Geometry: see drawing. Coordinates: mm, zero at the bounding-box minimum. Round coordinates to 2 decimals unless told otherwise and drop trailing zeros. Order: outer loops, then holes, each group sorted by start corner. A loop starts at its lowest first (then second) coordinate and runs counter-clockwise, first axis right, second up. Notation, with made-up numbers: (30.25, 73.25) -> (36.25, 73.25) arc R22 ccw to (36.25, 108.25) -> close; hole circle Ø4 at (-13, 87). An arc over 180 degrees is marked (long way). Answer as CSV lines item,"result". Start each with the question number.
(1) Section query A-A (y = 0.9). Output: boundary loops of the cut face in (x, z).
(2) Section query B-B (x = 54). Output: boundary loops of the cut face in (y, z).
(3) Contact query for flat-ended pins moving along their axis: P1, Ø0.9, axis at y = 1, z = 81.5, coming from the +X side; P2, Ø1.5, axis at x = 55, y = 1.5, coming from the -Z side. Output: stop coordinate, or through.
(4) Section query C-C (z = 18.5). Output: boundary loops of the cut face in (x, y), plus the area to 3 significant figures.
(5) Line query: line 1 along Z through (x, y) = (55.5, 1.65); line 2 along X through (y, z) = (2.6, 14); line 3 along X through (y, z) = (0.2, 61.5) (3 decimals). Output: solid intervals per line, ascending. Write a range as from..to.
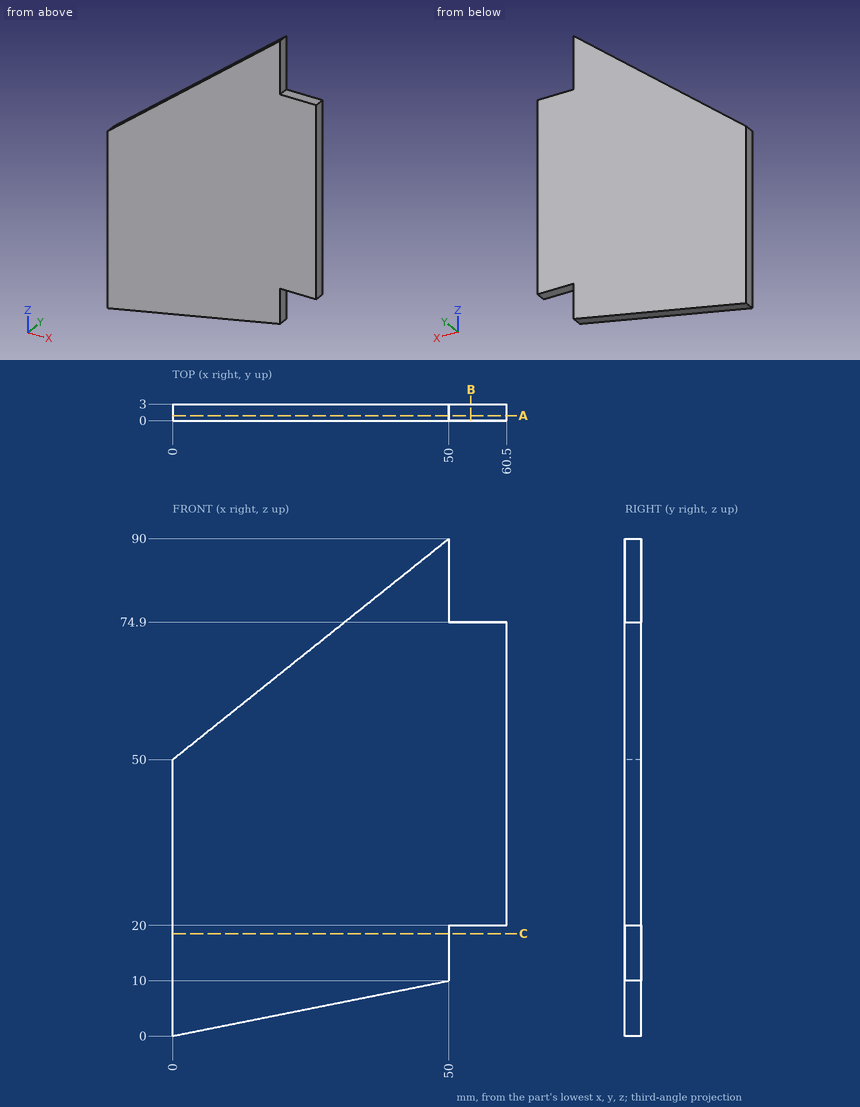
Answer block:
1,outline,"(0, 0) -> (50, 10) -> (50, 20) -> (60.5, 20) -> (60.5, 74.9) -> (50, 74.9) -> (50, 90) -> (0, 50) -> close"
2,outline,"(0, 20) -> (3, 20) -> (3, 74.9) -> (0, 74.9) -> close"
3,P1,"x = 50"
3,P2,"z = 20"
4,outline,"(0, 0) -> (50, 0) -> (50, 3) -> (0, 3) -> close"
4,area,"150 mm2"
5,line 1,"20..74.9"
5,line 2,"0..50"
5,line 3,"14.375..60.5"
